```python
from build123d import *

# Parameters (mm, degrees)
F0_R     = 2
F1_DEPTH = 3.5
F3_DEPTH = 50
F4_R     = 5
F5_DEPTH = 70.001


with BuildPart() as f1:
    # F0 (on Top) → F1 (new body)
    with BuildSketch(Plane.XY):
        Polygon((-10, -10), (-10, -60), (10, -60), (10, -10), (60, -10), (60, 10), (10, 10), (-10, 10), align=None)
        with Locations((0, -43)):
            Circle(F0_R, mode=Mode.SUBTRACT)
        with Locations((0, -24)):
            Circle(F0_R, mode=Mode.SUBTRACT)
        Circle(F0_R, mode=Mode.SUBTRACT)
        with Locations((24, 0)):
            Circle(F0_R, mode=Mode.SUBTRACT)
        with Locations((43, 0)):
            Circle(F0_R, mode=Mode.SUBTRACT)
    extrude(amount=F1_DEPTH)

    # F2 (on face) → F3 (join)
    with BuildSketch(Plane.XY.offset(3.5)):
        Polygon((8.289474, 10), (-10, 10), (-10, -8.289474), (-6.464466, -8.289474), (-6.464466, 6.464466), (8.289474, 6.464466), align=None)
    extrude(amount=F3_DEPTH)

    # F4 (on face) → F5 (cut, through all)
    with BuildSketch(Plane(origin=(-10, 0, 0), x_dir=(0, -1, 0), z_dir=(-1, 0, 0))):
        with Locations((-0.639477, 40.001725)):
            Circle(F4_R)
    extrude(amount=-F5_DEPTH, mode=Mode.SUBTRACT)


solid = f1.part
```
Build history of the part. All positions in model axes, mm. A direction names the side the tool comes from. Round coordinates to 2 decimals unless told otherwise and drop trailing zeros. Loops run counter-clockwise (first coordinate to the right, second up) from the corner with the lowest first, then second, coordinate; pieces in that order, holes last. Notation, with made-up numbers: M -24,70.5 L 27,70.5 A11 ccw 27,85.5 Z; hole C -13.75,4 d1. An arc over 180 degrees is marked long. Answer as CSV lines item,"result".
1. Cut at A-A on y = -43. Write the cut outline in (x, z).
Resolved:
outline,"M -10,0 L -2,0 L -2,3.5 L -10,3.5 Z; M 2,0 L 10,0 L 10,3.5 L 2,3.5 Z"
2. Two-plate mould, pull along Y, no slides. Class faces 4 (the cylindrical face through (22, 0, 2)), 5 (the flat face through (-7, 5, 53.5)), 6 (the flat face through (7, 10, 21)): released by +Y, released by -Y, zero draft, split by the parting line, or undercut.
Resolved:
face 4,"undercut"
face 5,"zero draft"
face 6,"released by +Y"
3. 3-axis set-ups, long thin cutter, end or side, ignore diameter. For faces 1 (the flat face through (1, 6.464, 28)), 2 (the flat face through (35, -10, 2)), 3 (the flat face through (-8, -8.289, 28)): which of +Z, -Z, +X, -X, +Y, -Y reach the whole face in a straight line?
Resolved:
face 1,"+Z, +X, -Y"
face 2,"+Z, -Z, +X, -Y"
face 3,"+Z, +X, -X, -Y"
4. Cut at D-D on z = 12. Write the cut outline in (x, y), then the cut area to 3 significant figures.
Resolved:
outline,"M -10,-8.29 L -6.46,-8.29 L -6.46,6.46 L 8.29,6.46 L 8.29,10 L -10,10 Z"
area,"117 mm²"
5. Wall check: probe 1 along Y at (x, z) = (0, 1); probe 2 along Y at (x, z) = (43, 2.05); probe 3 along Y at (x, z) = (-2, 16). Give the ranges that are in metal, low to high. Write a range as [from, to].
Resolved:
probe 1,"y = [-60, -45], [-41, -26], [-22, -2], [2, 10]"
probe 2,"y = [-10, -2], [2, 10]"
probe 3,"y = [6.46, 10]"
6. Flat gauge pins, fed straight in: P1, Ø16, axis at y = 0.64, z = 40, coming from the -X side; P2, Ø21, axis at x = 15, y = -12, coming from the +Z side; P3, Ø1.1, axis at x = -7.5, z = 35, coming from the -Y side; P4, Ø1.1, axis at y = 8, z = 39.5, coming from the +X side. Where does each tip first touch, or does it go through?
Resolved:
P1,"stops at x = -10"
P2,"stops at z = 3.5"
P3,"stops at y = -8.29"
P4,"stops at x = 8.29"
7. Cut at B-B on x = 0. Write the cut outline in (y, z), then the cut area to 3 significant figures.
Resolved:
outline,"M -60,0 L -45,0 L -45,3.5 L -60,3.5 Z; M -41,0 L -26,0 L -26,3.5 L -41,3.5 Z; M -22,0 L -2,0 L -2,3.5 L -22,3.5 Z; M 2,0 L 10,0 L 10,53.5 L 6.46,53.5 L 6.46,3.5 L 2,3.5 Z"
area,"380 mm²"
